Design review of the part built by this model. Coordinates are the model's own, in mm. A direction names the side the tool comes from. Round coordinates to 2 decimals unless told otherwise and drop trailing zeros. Loops run counter-clockwise (first coordinate to the right, second up) from the corner with the lowest first, then second, coordinate; pieces in that order, holes last. Notation, with made-up numbers: M -29.5,-32 L -14.5,-32 A20 cw -14.5,-1 Z; hole C 1,-8 d10. An arc over 180 degrees is marked long. One line per item, written item: value. Start each with the question number.
Item 1: We need section D-D (x = -28). Write out the cut boundary in (y, z), then the cut area to 3 significant figures.
Item 2: For line 1 along Z through (x, y) = (27, 1.5); line 2 along X through (y, z) = (1.2, 26); line 3 along X through (y, z) = (3.2, 0), list the stretches that pass through material, from the lowest coordinate up.
Item 3: We need section C-C (z = -18.75). Write out the cut boundary in (x, y), then the cut area to 3 significant figures.
Item 4: We need section B-B (x = 0). Write out the cut boundary in (y, z).
Item 5: For faces 1 (the cylindrical face through (29.038, 2.465, 27.996)), 2 (the flat face through (17, 2, -40.286)), 3 (the flat face through (0, 2, -35)), list the 3-axis set-ups (+Z, -Z, +X, -X, +Y, -Y) from which the entire face can be reached by the end or side of a thin tool; tool diameter is ignored.
Item 6: We need section A-A (y = 3.1). Write out the cut boundary in (x, z).
Item 7: Clearance check with flat-ended pins moving along their axes: pin 1 (6 mm diameter, centred on x = -28, z = 26, fed in from -Y); pin 2 (1 mm diameter, centred on x = -4.5, y = 3, fed in from +Z); pin 3 (2.5 mm diameter, centred on y = 2, z = -38.5, fed in from +X); pin 4 (1.5 mm diameter, centred on x = 5.5, y = 0.5, fed in from -Z). State where each tip first meets the part, or that it passes through.
Item 8: Mouldability with a two-part tool opening along X and no side actions: class faces 4 (the flat face through (1, 0, 20)), 5 (the cylindrical face through (-26.962, 2.465, 27.996)), 6 (the cylindrical face through (1.558, 2.465, 44.473)) as released by +X, released by -X, zero draft, split by the parting line, or undercut.
from build123d import *

# Parameters (mm, degrees)
SKETCH_2_R      = 15.25
SKETCH_2_R_2    = 2.25
EXTRUDE_1_DEPTH = 5


with BuildPart() as part:
    # Эскиз2 → Бобышка-Вытянуть1 (new body)
    with BuildSketch(Plane(origin=(0, 0, 0), x_dir=(1, 0, 0), z_dir=(0, 1, 0))):
        with BuildLine():
            Line((-15.5, 35), (15.5, 35))
            Line((15.5, 35), (15.5, 40.286336603))
            Line((15.5, 40.286336603), (18.901351356, 40.286336603))
            ThreePointArc((18.901351356, 40.286336603), (-0.126903456, -44.49981905), (-18.671270685, 40.393485254))
            Line((-18.671270685, 40.393485254), (-15.5, 40.393485254))
            Line((-15.5, 40.393485254), (-15.5, 35))
        make_face()
        Circle(SKETCH_2_R, mode=Mode.SUBTRACT)
        with Locations((-27, 18.75)):
            Circle(SKETCH_2_R_2, mode=Mode.SUBTRACT)
        with Locations((27, 18.75)):
            Circle(SKETCH_2_R_2, mode=Mode.SUBTRACT)
        with Locations((28, -26)):
            Circle(SKETCH_2_R_2, mode=Mode.SUBTRACT)
        with Locations((-28, -26)):
            Circle(SKETCH_2_R_2, mode=Mode.SUBTRACT)
    extrude(amount=EXTRUDE_1_DEPTH)


solid = part.part
A:
1. outline: M 0,-34.59 L 5,-34.59 L 5,-20.77 L 0,-20.77 Z; M 0,-16.73 L 5,-16.73 L 5,23.75 L 0,23.75 Z; M 0,28.25 L 5,28.25 L 5,34.59 L 0,34.59 Z
1. area: 303 mm2
2. line 1: -35.37 to -21, -16.5 to 23.98, 28.02 to 35.37
2. line 2: -36.11 to -30.25, -25.75 to 25.75, 30.25 to 36.11
2. line 3: -44.5 to -15.25, 15.25 to 44.5
3. outline: M -40.36,0 L -29.25,0 L -29.25,5 L -40.36,5 Z; M -24.75,0 L 24.75,0 L 24.75,5 L -24.75,5 Z; M 29.25,0 L 40.36,0 L 40.36,5 L 29.25,5 Z
3. area: 359 mm2
4. outline: M 0,-35 L 5,-35 L 5,-15.25 L 0,-15.25 Z; M 0,15.25 L 5,15.25 L 5,44.5 L 0,44.5 Z
5. face 1: +Y, -Y
5. face 2: -Z, +X, +Y, -Y
5. face 3: -Z, +Y, -Y
6. outline: M -18.67,-40.39 L -15.5,-40.39 L -15.5,-35 L 15.5,-35 L 15.5,-40.29 L 18.9,-40.29 A44.5 ccw long Z; hole C -28,26 d4.5; hole C -27,-18.75 d4.5; hole C 0,0 d30.5; hole C 27,-18.75 d4.5; hole C 28,26 d4.5
7. pin 1: y = 0
7. pin 2: z = 44.32
7. pin 3: x = 24.35
7. pin 4: z = -35
8. face 4: zero draft
8. face 5: undercut
8. face 6: split by the parting line
